```python
from build123d import *

# Parameters (mm, degrees)
SKETCH020_R     = 1.6
PAD015_DEPTH    = 15
SKETCH021_R     = 3.5
PAD016_DEPTH    = 3
SKETCH022_R     = 1.75
POCKET003_DEPTH = 2
FILLET002_R     = 1


with BuildPart() as part:
    # Sketch020 → Pad015 (new body)
    with BuildSketch(Plane.XY):
        with Locations((-72.372711, 11.675275)):
            Circle(SKETCH020_R)
    extrude(amount=PAD015_DEPTH)

    # Sketch021 → Pad016 (join)
    with BuildSketch(Plane.XY):
        with Locations((-72.372711, 11.675275)):
            Circle(SKETCH021_R)
    extrude(amount=-PAD016_DEPTH)

    # Sketch022 (on Face3 of Pad016) → Pocket003 (cut)
    with BuildSketch(Plane(origin=(0, 0, -3), x_dir=(1, 0, 0), z_dir=(0, 0, -1))):
        with Locations((-72.372711, -11.675275)):
            Circle(SKETCH022_R)
    extrude(amount=-POCKET003_DEPTH, mode=Mode.SUBTRACT)

    # Fillet002
    fillet002_edges = [part.edges().sort_by_distance(p)[0] for p in [
        (-73.972711, 11.675275, 0),
    ]]
    fillet(fillet002_edges, radius=FILLET002_R)


solid = part.part
```
Design review of the part built by this model. Coordinates are the model's own, in mm. A direction names the side the tool comes from. Coordinates: 2 decimals unless noted, no trailing zeros. Loops run counter-clockwise (first coordinate to the right, second up) from the corner with the lowest first, then second, coordinate; pieces in that order, holes last.
Q1. We need section A-A on y = 14.5. State the section outline as (x, z) points.
Reported:
outline: (-74.44, -3) - (-70.31, -3) - (-70.31, 0) - (-74.44, 0) - close
Q2. To check wall thickness, follow line 1 (Z direction, x = -69.75, y = 9.5); line 2 (X direction, y = 10.5, z = -2.25); line 3 (Y direction, x = -71.5, z = 6.75). State the ranges of each line that lie inside material, in increasing order.
Reported:
line 1: z = -3 to 0
line 2: x = -75.67 to -73.67, -71.08 to -69.08
line 3: y = 10.33 to 13.02
Q3. For pin 1 (2 mm diameter, centred on x = -71.5, z = 2, fed in from -Y); pin 2 (2 mm diameter, centred on x = -72.37, y = 11.68, fed in from -Z); pin 3 (1.5 mm diameter, centred on x = -72.5, z = 0, fed in from -Y), all flat-tipped, find the tip position at first contact; note any pin that passes through.
Reported:
pin 1: stops at y = 10.08
pin 2: stops at z = -1
pin 3: stops at y = 8.18
Q4. We need section B-B on z = 10. State the section outline as (x, y) points.
Reported:
outline: circle Ø3.2 at (-72.37, 11.68)
Q5. We need section C-C on x = -75.5. State the section outline as (y, z) points, and give its area (3 significant figures).
Reported:
outline: (10.1, -3) - (13.25, -3) - (13.25, 0) - (10.1, 0) - close
area: 9.43 mm2
Q6. The part is to be moulded in two halves that separate along Y. For faces 1 (the face through (-70.704, 11.15, -2.014)), 2 (the face through (-75, 10, 0)), 3 (the face through (-72, 12, -1)), 4 (the face through (-70.491, 14.626, -1.479)), say which applies: +Y half, -Y half, draft (parallel to the pull), parting line (faces both ways), or undercut.
Reported:
face 1: undercut
face 2: draft
face 3: undercut
face 4: parting line
Q7. Tool access review of faces 5 (the face through (-72, 12, 15)), 6 (the face through (-70.895, 11.062, 7.902)): name each direction out of +Z, -Z, +X, -X, +Y, -Y from which nothing blocks a thin tool from reaching the whole face with its end or side.
Reported:
face 5: +Z, +X, -X, +Y, -Y
face 6: +Z
